Verification items for the finished model (mm, model axes). Give positions to 0.01 mm unless a question says otherwise; leave off trailing zeros. Order: outer loops, then holes, each group sorted by start corner. A loop starts at its lowest first (then second) coordinate and runs counter-clockwise, first axis right, second up.
(1) Gauge pin test, flat ends, axial feed: pin 1 (4 mm diameter, centred on x = 15, y = 9.5, fed in from +Z); pin 2 (1.5 mm diameter, centred on y = 7.5, z = 22.5, fed in from +X); pin 3 (8 mm diameter, centred on y = -17.5, z = 20, fed in from +X). Record the tip position at first contact, or that the pin passes through.
(2) Scan lines: L1, parallel to Z at x = 0.5, y = -12; L2, parallel to Z at x = -28, y = -8; L3, parallel to Y at x = 10.5, z = 15.5. Record each from-to range of solid material in increasing order.
(3) Sectioned sample at D-D on z = 17.5. Record the cut outline in (x, y).
(4) Sectioned sample at C-C on z = 33. Record the cut outline in (x, y), plus the area to 3 significant figures.
(5) Sectioned sample at A-A on y = 0. Record the cut outline in (x, z).
```python
from build123d import *

# Parameters (mm, degrees)
F0_R     = 32.7640800534
F1_DEPTH = 38.1
F2_SIZE  = 22.86
F3_SIZE  = 5.08


# Not quite as in the source:
# - a fillet or chamfer that OpenCascade refuses, or shapes differently, is made with other operations: its cross-section is extruded or revolved along the edge and cut away or added


with BuildPart() as f1:
    # F0 (on Top) → F1 (new body)
    with BuildSketch(Plane.XY):
        Circle(F0_R)
    extrude(amount=F1_DEPTH)

    # F2
    f2_edges = [f1.edges().sort_by_distance(p)[0] for p in [
        (-32.76408, 0, 38.1),
    ]]
    chamfer(f2_edges, length=F2_SIZE)

    # F3
    f3_edges = [f1.edges().sort_by_distance(p)[0] for p in [
        (-32.76408, 0, 0),
    ]]
    chamfer(f3_edges, length=F3_SIZE)

    # F4: chamfer of 22.86 on 1 edges, made by hand

    # F4_s1 → F4_t2 (revolve, cut)
    with BuildSketch(Plane.XZ):
        Polygon((43.8485410713, 16.1644610179), (4.8240800534, 0), (27.6840800534, 0), align=None)
    revolve(axis=Axis((0, 0, 0), (0, 0, 1)), mode=Mode.SUBTRACT)


solid = f1.part
```
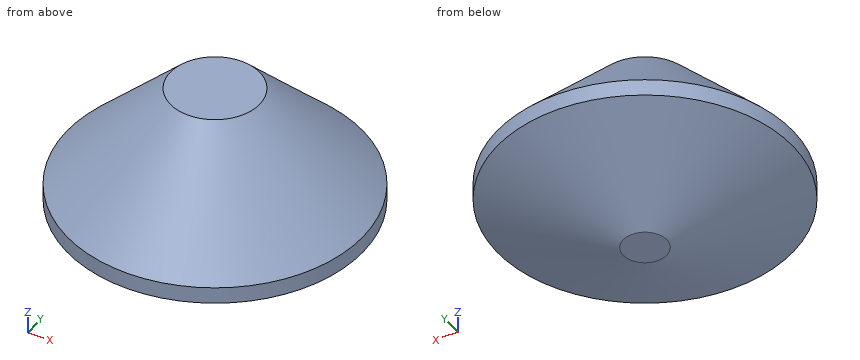
Ans:
1. pin 1: stops at z = 32.25
1. pin 2: stops at x = 25.19
1. pin 3: stops at x = 27.4
2. L1: z = 2.98 to 35.99
2. L2: z = 10.06 to 18.88
2. L3: y = -30.76 to 30.76
3. outline: circle Ø61.01 at (0, 0)
4. outline: circle Ø30.01 at (0, 0)
4. area: 707 mm2
5. outline: (-32.76, 11.57) - (-4.82, 0) - (4.82, 0) - (32.76, 11.57) - (32.76, 15.24) - (9.9, 38.1) - (-9.9, 38.1) - (-32.76, 15.24) - close
